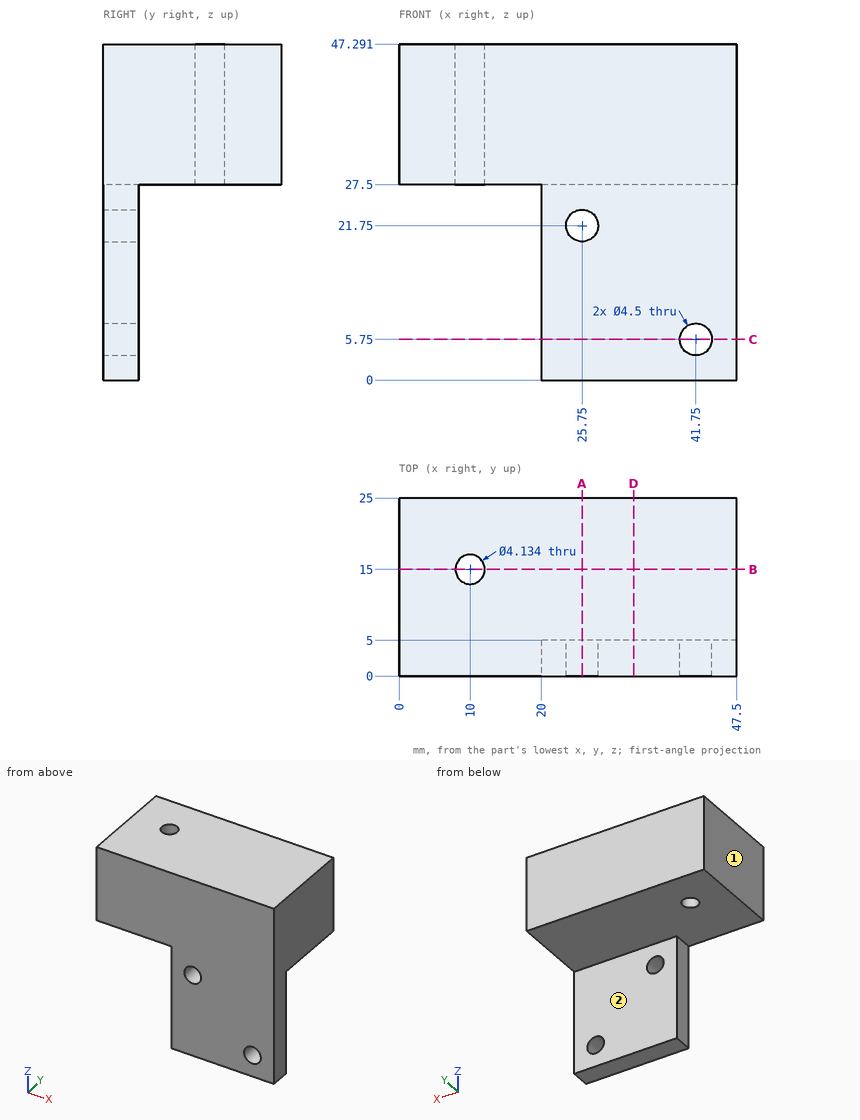
Study the drawing (mm; zero at the part's minimum x, y, z) and answer. A direction names the side the tool comes from. Coordinates: 2 decimals unless noted, no trailing zeros. Loops run counter-clockwise (first coordinate to the right, second up) from the corner with the lowest first, then second, coordinate; pieces in that order, holes last. Notation, with made-up numbers: (54.5, -28) -> (69.5, -28) arc R17 cw to (69.5, -12) -> close; hole circle Ø5 at (85, 49). An arc over 180 degrees is marked (long way). Write each question's results on one line, items separated by ' | '. Start each with the question number.
1) Flat-ended cylindrical pins translate along their axes: P1, Ø8, axis at x = 29.5, z = 15.5, coming from the +Y side; P2, Ø3, axis at x = 35.5, y = 11, coming from the -Z side; P3, Ø4, axis at y = 3.5, z = 7.5, coming from the -X side. Find the tip coordinate at first contact, or state that the pin passes through.
2) For the marked faces 1 and 2, determine the directions among +Z, -Z, +X, -X, +Y, -Y from which every point of the face is accessible in a straight line to the end or side of a thin tool.
3) Find section A-A on x = 25.75. Determine the outline of the cut face in (y, z), then the cut area to 3 significant figures.
4) Find section C-C on z = 5.75. Determine the outline of the cut face in (x, y).
5) Consider line 1 along Y through (x, z) = (10, 40); line 2 along X through (y, z) = (15, 34.25); line 3 along Z through (x, y) = (41.75, 3.1). Determine where each line is inside the solid, lowest interval first.
6) Find section D-D on x = 33. Determine the outline of the cut face in (y, z), then the cut area to 3 significant figures.
7) Find section B-B on y = 15. Determine the outline of the cut face in (x, z), then the cut area to 3 significant figures.
Response values:
1) P1: stops at y = 5 | P2: stops at z = 27.5 | P3: stops at x = 20
2) face 1: +Z, -Z, -X, +Y, -Y | face 2: -Z, +X, -X, +Y
3) outline: (0, 0) -> (5, 0) -> (5, 19.5) -> (0, 19.5) -> close; (0, 24) -> (5, 24) -> (5, 27.5) -> (25, 27.5) -> (25, 47.29) -> (0, 47.29) -> close | area: 610 mm^2
4) outline: (20, 0) -> (39.5, 0) -> (39.5, 5) -> (20, 5) -> close; (44, 0) -> (47.5, 0) -> (47.5, 5) -> (44, 5) -> close
5) line 1: y = 0 to 12.93, 17.07 to 25 | line 2: x = 0 to 7.93, 12.07 to 47.5 | line 3: z = 0 to 3.5, 8 to 47.29
6) outline: (0, 0) -> (5, 0) -> (5, 27.5) -> (25, 27.5) -> (25, 47.29) -> (0, 47.29) -> close | area: 632 mm^2
7) outline: (0, 27.5) -> (7.93, 27.5) -> (7.93, 47.29) -> (0, 47.29) -> close; (12.07, 27.5) -> (47.5, 27.5) -> (47.5, 47.29) -> (12.07, 47.29) -> close | area: 858 mm^2
